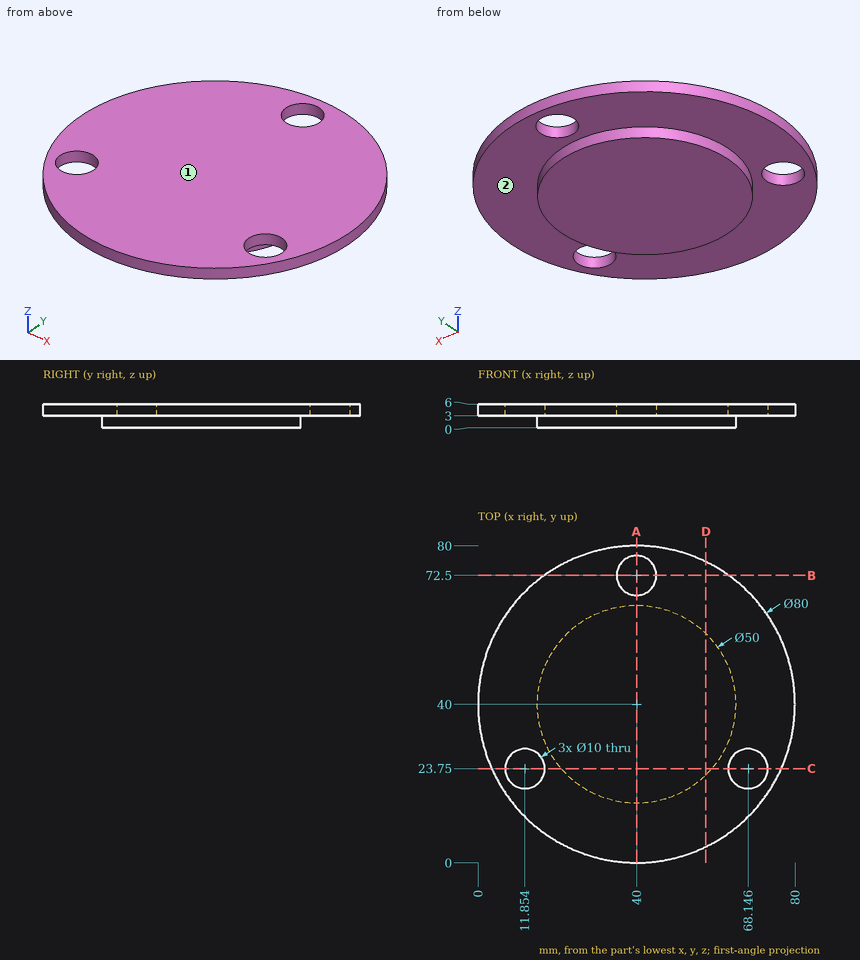
Study the drawing (mm; zero at the part's minimum x, y, z) and answer. A direction names the side the tool comes from. Give positions to 0.01 mm unless a question says otherwise; leave off trailing zeros. Loops run counter-clockwise (first coordinate to the right, second up) from the corner with the lowest first, then second, coordinate; pieces in that order, holes last. Notation, with made-up numbers: M 22,24 L 39,24 A24 cw 39,56 Z; hole C 50.25,69.25 d1. An arc over 180 degrees is marked long. Use CSV: the item, a comma, the result in double quotes.
1) Find section B-B on y = 72.5. Write down the section's boundary in (x, z).
Answer:
outline,"M 16.68,3 L 35,3 L 35,6 L 16.68,6 Z; M 45,3 L 63.32,3 L 63.32,6 L 45,6 Z"
2) Given P1, Ø3, axis at x = 11.5, z = 4.5, coming from the +Y side; P2, Ø1, axis at y = 49, z = 4, coming from the -X side; P3, Ø13, axis at x = 40, y = 72.5, coming from the -Z side, each flat-ended and moving along its own axis, determine where each tip first touches the part or whether it passes through.
Answer:
P1,"y = 69.51"
P2,"x = 0.91"
P3,"z = 3"
3) Consider L1, parallel to Z at x = 15.5, y = 47; L2, parallel to Y at x = 40, z = 4.7; L3, parallel to Y at x = 66, z = 4.45. Determine where each line is inside the solid, lowest interval first.
Answer:
L1,"3 to 6"
L2,"0 to 67.5, 77.5 to 80"
L3,"9.6 to 19.23, 28.27 to 70.4"
4) Find section A-A on x = 40. Write down the section's boundary in (y, z), plus the area to 3 significant figures.
Answer:
outline,"M 0,3 L 15,3 L 15,0 L 65,0 L 65,3 L 67.5,3 L 67.5,6 L 0,6 Z; M 77.5,3 L 80,3 L 80,6 L 77.5,6 Z"
area,"360 mm^2"
5) Which of the six approach directions +Z, -Z, +X, -X, +Y, -Y give full straight-line access (tool end or side, diameter ignored) to the marked faces 1 and 2?
Answer:
face 1,"+Z, +X, -X, +Y, -Y"
face 2,"-Z"
6) Find section D-D on x = 57.5. Write down the section's boundary in (y, z), plus the area to 3 significant figures.
Answer:
outline,"M 4.03,3 L 22.15,3 L 22.15,0 L 57.85,0 L 57.85,3 L 75.97,3 L 75.97,6 L 4.03,6 Z"
area,"323 mm^2"
7) Find section C-C on y = 23.75. Write down the section's boundary in (x, z).
Answer:
outline,"M 3.45,3 L 6.85,3 L 6.85,6 L 3.45,6 Z; M 16.85,3 L 21,3 L 21,0 L 59,0 L 59,3 L 63.15,3 L 63.15,6 L 16.85,6 Z; M 73.15,3 L 76.55,3 L 76.55,6 L 73.15,6 Z"
